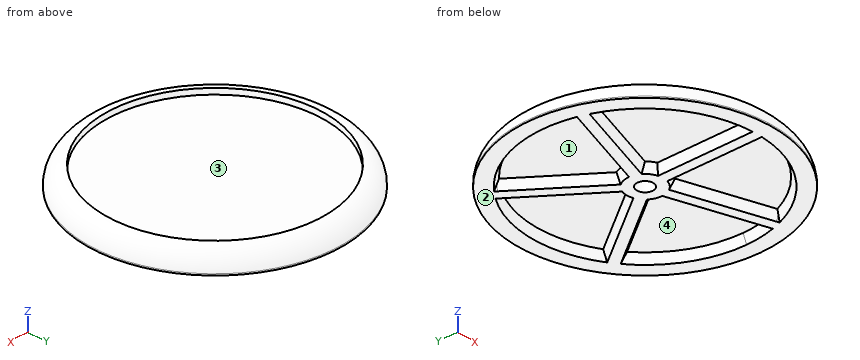
```python
from build123d import *

# Parameters (mm, degrees)
F0_R     = 25
F0_R_2   = 21.5
F1_DEPTH = 3.8
F2_DEPTH = 2.66
F3_R     = 3.49999
F4_R     = 1.6
F5_DEPTH = 1.9
F6_DEPTH = 1.66
F6_TAPER = 25


# Not quite as in the source:
# - a fillet or chamfer is up to 0.001 mm smaller than in the source, because OpenCascade refuses the exact size


with BuildPart() as f1:
    # F0 (on Top) → F1 (new body)
    with BuildSketch(Plane.XY):
        Circle(F0_R)
        Circle(F0_R_2, mode=Mode.SUBTRACT)
    extrude(amount=F1_DEPTH)

    # F0 (on Top) → F2 (join, through all)
    with BuildSketch(Plane.XY):
        Circle(F0_R_2)
    extrude(amount=F2_DEPTH)

    # F3 (radius 3.5 in the source; OpenCascade refuses exactly that, so slightly less here)
    f3_edges = [f1.edges().sort_by_distance(p)[0] for p in [
        (-25, 0, 3.8),
    ]]
    fillet(f3_edges, radius=F3_R)

    # F4 (on face) → F5 (cut)
    with BuildSketch(Plane.XY):
        Circle(F4_R)
    extrude(amount=F5_DEPTH, mode=Mode.SUBTRACT)

    # F4 (on face) → F6 (cut, through all)
    with BuildSketch(Plane.XY):
        with BuildLine():
            Line((-1, -21.4767315949), (-1, -3.4583232932))
            ThreePointArc((-1, -3.4583232932), (-2.1160269083, -2.9124611797), (-2.980043909, -2.0197371859))
            Line((-2.980043909, -2.0197371859), (-20.1165685377, -7.5877315628))
            ThreePointArc((-20.1165685377, -7.5877315628), (-12.6373829243, -17.3938653791), (-1, -21.4767315949))
        make_face()
        with BuildLine():
            Line((-1, -21.9772609758), (-1, -21.4767315949))
            ThreePointArc((-1, -21.4767315949), (-12.6373829243, -17.3938653791), (-20.1165685377, -7.5877315628))
            Line((-20.1165685377, -7.5877315628), (-20.592600267, -7.7424036476))
            ThreePointArc((-20.592600267, -7.7424036476), (-12.9312755504, -17.7983738762), (-1, -21.9772609758))
        make_face()
        with BuildLine():
            Line((20.1165685377, -7.5877315628), (2.980043909, -2.0197371859))
            ThreePointArc((2.980043909, -2.0197371859), (2.1160269083, -2.9124611797), (1, -3.4583232932))
            Line((1, -3.4583232932), (1, -21.4767315949))
            ThreePointArc((1, -21.4767315949), (12.6373829243, -17.3938653791), (20.1165685377, -7.5877315628))
        make_face()
        with BuildLine():
            Line((20.592600267, -7.7424036476), (20.1165685377, -7.5877315628))
            ThreePointArc((20.1165685377, -7.5877315628), (12.6373829243, -17.3938653791), (1, -21.4767315949))
            Line((1, -21.4767315949), (1, -21.9772609758))
            ThreePointArc((1, -21.9772609758), (12.9312755504, -17.7983738762), (20.592600267, -7.7424036476))
        make_face()
        with BuildLine():
            ThreePointArc((2.8417684238, 2.2100570639), (3.4051700637, 1.1682537555), (3.6, 0))
            ThreePointArc((3.6, 0), (3.5995194424, -0.0588199284), (3.5980778978, -0.1176241533))
            Line((3.5980778978, -0.1176241533), (20.7346025264, -5.6856185302))
            ThreePointArc((20.7346025264, -5.6856185302), (21.307791466, -2.8684530397), (21.5, 0))
            ThreePointArc((21.5, 0), (19.3785131848, 9.3125306307), (13.4327230933, 16.7872555916))
            Line((13.4327230933, 16.7872555916), (2.8417684238, 2.2100570639))
        make_face()
        with BuildLine():
            Line((13.7269268818, 17.192192367), (13.4327230933, 16.7872555916))
            ThreePointArc((13.4327230933, 16.7872555916), (19.3785131848, 9.3125306307), (21.5, 0))
            ThreePointArc((21.5, 0), (21.307791466, -2.8684530397), (20.7346025264, -5.6856185302))
            Line((20.7346025264, -5.6856185302), (21.2106342558, -5.8402906151))
            ThreePointArc((21.2106342558, -5.8402906151), (21.8017654518, -2.9466969961), (22, 0))
            ThreePointArc((22, 0), (19.8241316506, 9.5395914116), (13.7269268818, 17.192192367))
        make_face()
        with BuildLine():
            ThreePointArc((-1.223734435, 3.3856275685), (0, 3.6), (1.223734435, 3.3856275685))
            Line((1.223734435, 3.3856275685), (11.8146891046, 17.9628260962))
            ThreePointArc((11.8146891046, 17.9628260962), (0, 21.5), (-11.8146891046, 17.9628260962))
            Line((-11.8146891046, 17.9628260962), (-1.223734435, 3.3856275685))
        make_face()
        with BuildLine():
            ThreePointArc((-11.8146891046, 17.9628260962), (0, 21.5), (11.8146891046, 17.9628260962))
            Line((11.8146891046, 17.9628260962), (12.108892893, 18.3677628716))
            ThreePointArc((12.108892893, 18.3677628716), (0, 22), (-12.108892893, 18.3677628716))
            Line((-12.108892893, 18.3677628716), (-11.8146891046, 17.9628260962))
        make_face()
        with BuildLine():
            ThreePointArc((-3.5980778978, -0.1176241533), (-3.4238034587, 1.1124611797), (-2.8417684238, 2.2100570639))
            Line((-2.8417684238, 2.2100570639), (-13.4327230933, 16.7872555916))
            ThreePointArc((-13.4327230933, 16.7872555916), (-20.4477151003, 6.6438653791), (-20.7346025264, -5.6856185302))
            Line((-20.7346025264, -5.6856185302), (-3.5980778978, -0.1176241533))
        make_face()
        with BuildLine():
            ThreePointArc((-20.7346025264, -5.6856185302), (-20.4477151003, 6.6438653791), (-13.4327230933, 16.7872555916))
            Line((-13.4327230933, 16.7872555916), (-13.7269268818, 17.192192367))
            ThreePointArc((-13.7269268818, 17.192192367), (-20.9232433585, 6.7983738762), (-21.2106342558, -5.8402906151))
            Line((-21.2106342558, -5.8402906151), (-20.7346025264, -5.6856185302))
        make_face()
    extrude(amount=F6_DEPTH, taper=F6_TAPER, mode=Mode.SUBTRACT)


solid = f1.part
```
Input: part model. Units: mm. Frame: model coordinates. Face numbers are marked on the shaded views. A direction names the side the tool comes from. Give positions to 0.01 mm unless a question says otherwise; leave off trailing zeros. Use a Markdown table: item, result.
(1) Access query for the marked faces 3 and 4. Directions: +Z, -Z, +X, -X, +Y, -Y. A direction counts if a zero-diameter tool reaches every point of the face in a straight line with its end or side. Return the directions, or none.
Computed values:
| item | result |
|---|---|
| face 3 | +Z |
| face 4 | -Z |
(2) Draft query along Y for the marked faces 1 and 2. Return one class per face: released by +Y, released by -Y, zero draft, split by the parting line, or undercut.
Computed values:
| item | result |
|---|---|
| face 1 | undercut |
| face 2 | zero draft |
(3) Line query: line 1 (Y direction, x = -15.5, z = 0.75); line 2 (Y direction, x = 0, z = 1.2); line 3 (Y direction, x = -10, z = 0.9). Output: solid intervals per line, ascending. Write a range as from..to.
Computed values:
| item | result |
|---|---|
| line 1 | y = -19.58..-15.12, -6.46..-3.62, 15.12..19.58 |
| line 2 | y = -24.88..-1.6, 1.6..4.16, 21.44..24.88 |
| line 3 | y = -22.86..-19.12, -4.74..-1.76, 11.35..16.18, 19.12..22.86 |
(4) Pin query (flat end, axial travel): pin 1 (1.5 mm diameter, centred on x = -10, y = -18, fed in from -Z); pin 2 (1 mm diameter, centred on x = -0.5, y = -0.5, fed in from -Z); pin 3 (13 mm diameter, centred on x = 2.5, y = -4.5, fed in from +Z). Return the tip coordinate at first contact, or that it passes through.
Computed values:
| item | result |
|---|---|
| pin 1 | stops at z = 1.41 |
| pin 2 | stops at z = 1.9 |
| pin 3 | stops at z = 2.66 |
